```python
from build123d import *

# Parameters (mm, degrees)
F0_R     = 31.9884370587
F1_DEPTH = 25.4


with BuildPart() as f1:
    # F0 (on Front) → F1 (new body)
    with BuildSketch(Plane.XZ):
        Circle(F0_R)
        with BuildLine():
            add(Edge.make_bspline(
                [(-4.1474287559, -5.2462848568), (-2.9695766051, -6.4846808097), (-2.9695766051, -8.3615386761)],
                knots=[0, 0, 0, 1, 1, 1], degree=2))
            add(Edge.make_bspline(
                [(-2.9695766051, -8.3615386761), (-2.9695766051, -10.9924420782), (-4.9289942017, -12.4207254106)],
                knots=[0, 0, 0, 1, 1, 1], degree=2))
            add(Edge.make_bspline(
                [(-4.9289942017, -12.4207254106), (-6.8884117983, -13.8490087429), (-10.4329762146, -13.8490087429)],
                knots=[0, 0, 0, 1, 1, 1], degree=2))
            add(Edge.make_bspline(
                [(-10.4329762146, -13.8490087429), (-14.1811879653, -13.8490087429), (-16.2782051122, -12.6601486281)],
                knots=[0, 0, 0, 1, 1, 1], degree=2))
            Line((-16.2782051122, -12.6601486281), (-16.2782051122, -10.0127332799))
            add(Edge.make_bspline(
                [(-16.2782051122, -10.0127332799), (-14.9187215551, -10.7007310315), (-13.3638466364, -11.0942657455)],
                knots=[0, 0, 0, 1, 1, 1], degree=2))
            add(Edge.make_bspline(
                [(-13.3638466364, -11.0942657455), (-11.8089717178, -11.4878004594), (-10.3614244484, -11.4878004594)],
                knots=[0, 0, 0, 1, 1, 1], degree=2))
            add(Edge.make_bspline(
                [(-10.3614244484, -11.4878004594), (-8.1268077512, -11.4878004594), (-6.9241876814, -10.7750347887)],
                knots=[0, 0, 0, 1, 1, 1], degree=2))
            add(Edge.make_bspline(
                [(-6.9241876814, -10.7750347887), (-5.7215676115, -10.0622691181), (-5.7215676115, -8.5982099026)],
                knots=[0, 0, 0, 1, 1, 1], degree=2))
            add(Edge.make_bspline(
                [(-5.7215676115, -8.5982099026), (-5.7215676115, -7.4974135001), (-6.6737564998, -6.7158480542)],
                knots=[0, 0, 0, 1, 1, 1], degree=2))
            add(Edge.make_bspline(
                [(-6.6737564998, -6.7158480542), (-7.625945388, -5.9342826084), (-10.3999523225, -4.8665100979)],
                knots=[0, 0, 0, 1, 1, 1], degree=2))
            add(Edge.make_bspline(
                [(-10.3999523225, -4.8665100979), (-13.0308557246, -3.8868012996), (-14.1399081002, -3.1547716919)],
                knots=[0, 0, 0, 1, 1, 1], degree=2))
            add(Edge.make_bspline(
                [(-14.1399081002, -3.1547716919), (-15.2489604758, -2.4227420842), (-15.7911027041, -1.495321115)],
                knots=[0, 0, 0, 1, 1, 1], degree=2))
            add(Edge.make_bspline(
                [(-15.7911027041, -1.495321115), (-16.3332449324, -0.5679001459), (-16.3332449324, 0.7200316452)],
                knots=[0, 0, 0, 1, 1, 1], degree=2))
            add(Edge.make_bspline(
                [(-16.3332449324, 0.7200316452), (-16.3332449324, 3.0262001086), (-14.456387066, 4.3609157467)],
                knots=[0, 0, 0, 1, 1, 1], degree=2))
            add(Edge.make_bspline(
                [(-14.456387066, 4.3609157467), (-12.5795291996, 5.6956313848), (-9.3156678659, 5.6956313848)],
                knots=[0, 0, 0, 1, 1, 1], degree=2))
            add(Edge.make_bspline(
                [(-9.3156678659, 5.6956313848), (-6.2719658128, 5.6956313848), (-3.360359328, 4.4572354319)],
                knots=[0, 0, 0, 1, 1, 1], degree=2))
            Line((-3.360359328, 4.4572354319), (-4.3785960004, 2.1345550225))
            add(Edge.make_bspline(
                [(-4.3785960004, 2.1345550225), (-7.213146737, 3.3013992092), (-9.5193152004, 3.3013992092)],
                knots=[0, 0, 0, 1, 1, 1], degree=2))
            add(Edge.make_bspline(
                [(-9.5193152004, 3.3013992092), (-11.5502845632, 3.3013992092), (-12.5822811906, 2.6656892867)],
                knots=[0, 0, 0, 1, 1, 1], degree=2))
            add(Edge.make_bspline(
                [(-12.5822811906, 2.6656892867), (-13.614277818, 2.0299793642), (-13.614277818, 0.9126710156)],
                knots=[0, 0, 0, 1, 1, 1], degree=2))
            add(Edge.make_bspline(
                [(-13.614277818, 0.9126710156), (-13.614277818, 0.1531214978), (-13.2262470861, -0.3780127664)],
                knots=[0, 0, 0, 1, 1, 1], degree=2))
            add(Edge.make_bspline(
                [(-13.2262470861, -0.3780127664), (-12.8382163542, -0.9091470306), (-11.9795951602, -1.3907454568)],
                knots=[0, 0, 0, 1, 1, 1], degree=2))
            add(Edge.make_bspline(
                [(-11.9795951602, -1.3907454568), (-11.1209739662, -1.8723438829), (-8.6772059525, -2.786004897)],
                knots=[0, 0, 0, 1, 1, 1], degree=2))
            add(Edge.make_bspline(
                [(-8.6772059525, -2.786004897), (-5.3252809066, -4.0078889039), (-4.1474287559, -5.2462848568)],
                knots=[0, 0, 0, 1, 1, 1], degree=2))
        make_face(mode=Mode.SUBTRACT)
        with BuildLine():
            Line((17.4336847166, -13.5022578761), (14.5771180519, -13.5022578761))
            Line((14.5771180519, -13.5022578761), (14.5771180519, -1.3054337356))
            add(Edge.make_bspline(
                [(14.5771180519, -1.3054337356), (14.5771180519, 0.9952307458), (13.5286094785, 2.1318030315)],
                knots=[0, 0, 0, 1, 1, 1], degree=2))
            add(Edge.make_bspline(
                [(13.5286094785, 2.1318030315), (12.480100905, 3.2683753171), (10.2399802258, 3.2683753171)],
                knots=[0, 0, 0, 1, 1, 1], degree=2))
            add(Edge.make_bspline(
                [(10.2399802258, 3.2683753171), (7.2678299388, 3.2683753171), (5.9000904086, 1.6502046053)],
                knots=[0, 0, 0, 1, 1, 1], degree=2))
            add(Edge.make_bspline(
                [(5.9000904086, 1.6502046053), (4.5323508784, 0.0320338936), (4.5323508784, -3.644626091)],
                knots=[0, 0, 0, 1, 1, 1], degree=2))
            Line((4.5323508784, -3.644626091), (4.5323508784, -13.5022578761))
            Line((4.5323508784, -13.5022578761), (1.6757842138, -13.5022578761))
            Line((1.6757842138, -13.5022578761), (1.6757842138, 13.2636066525))
            Line((1.6757842138, 13.2636066525), (4.5323508784, 13.2636066525))
            Line((4.5323508784, 13.2636066525), (4.5323508784, 5.1617451295))
            add(Edge.make_bspline(
                [(4.5323508784, 5.1617451295), (4.5323508784, 3.6976859141), (4.3947513281, 2.7344890619)],
                knots=[0, 0, 0, 1, 1, 1], degree=2))
            Line((4.3947513281, 2.7344890619), (4.5653747705, 2.7344890619))
            add(Edge.make_bspline(
                [(4.5653747705, 2.7344890619), (5.4074840185, 4.0939726191), (6.9651109281, 4.8755380649)],
                knots=[0, 0, 0, 1, 1, 1], degree=2))
            add(Edge.make_bspline(
                [(6.9651109281, 4.8755380649), (8.5227378378, 5.6571035107), (10.5151793264, 5.6571035107)],
                knots=[0, 0, 0, 1, 1, 1], degree=2))
            add(Edge.make_bspline(
                [(10.5151793264, 5.6571035107), (13.9716800305, 5.6571035107), (15.7026823736, 4.0141648799)],
                knots=[0, 0, 0, 1, 1, 1], degree=2))
            add(Edge.make_bspline(
                [(15.7026823736, 4.0141648799), (17.4336847166, 2.371226249), (17.4336847166, -1.2063620593)],
                knots=[0, 0, 0, 1, 1, 1], degree=2))
            Line((17.4336847166, -1.2063620593), (17.4336847166, -13.5022578761))
        make_face(mode=Mode.SUBTRACT)
    extrude(amount=F1_DEPTH)


solid = f1.part
```
Here's how the part is built. I have some questions about the finished solid (model axes, mm). A direction names the side the tool comes from. Give positions to 0.01 mm unless a question says otherwise; leave off trailing zeros. Order: outer loops, then holes, each group sorted by start corner. A loop starts at its lowest first (then second) coordinate and runs counter-clockwise, first axis right, second up. Notation, with made-up numbers: (8, 79.25) - (15, 79.25) arc R22 ccw to (15, 99.25) - close; hole circle Ø2 at (63.5, -11). An arc over 180 degrees is marked (long way). Answer as a JSON object with one key per item and string values. Group by question number.
Item 1: If we section it at D-D on x = -19: Please give me the cut outline in (y, z).
Item 2: If we section it at B-B on y = -19: Give the number of separate pieces and of enclosed holes in the cut face, and give its area (3 significant figures).
Item 3: Please list where these lines run through material, in increasing order: probe 1 along X at (y, z) = (-2, -9); probe 2 along Z at (x, y) = (-4, -3.75); probe 3 along Z at (x, y) = (-1, -7.75).
Item 4: If we section it at C-C on z = 19: Please give me the cut outline in (x, y), and give its area (3 significant figures).
Item 5: For P1, Ø6.5, axis at y = -15, z = 8, coming from the -X side; P2, Ø3, axis at x = -1, y = -3, coming from the +Z side; P3, Ø8, axis at x = -19, y = -13, coming from the -Z side, each with a flat end and sliding along its axis, tell me the tip position at first contact or that it passes through.
Item 6: If we mould it in two halves opening along Z, with no side actions, what happens to faces 3 (the flat face through (-4, -13, 3)), 4 (the cylindrical face through (-6.93, -12.52, -31.23)), 5 (the flat face through (0, -25.4, 0))? For each: pulls with the +Z half, pulls with the -Z half, needs draft (parallel to the pull), parting line crosses it, or undercut.
Item 7: Which directions (+Z, -Z, +X, -X, +Y, -Y) give clear straight access to the entire face, cutting with the end or side of a thin tool? Please do faces 1 (the flat face through (0, 0, 0)), 2 (the flat face through (3, -13, -13.502)).
Item 8: If we section it at A-A on z = 8: Please give me the cut outline in (x, y), and give its area (3 significant figures).
Result set:
{
 "1": {"outline": "(-25.4, -25.73) - (0, -25.73) - (0, 25.73) - (-25.4, 25.73) - close"},
 "2": {"separate pieces": "1", "enclosed holes": "2", "area": "2,950 mm²"},
 "3": {"probe 1": "-30.7 to -5.75, -3 to 1.68, 4.53 to 14.58, 17.43 to 30.7", "probe 2": "-31.74 to -11.54, -5.41 to 3, 4.71 to 31.74", "probe 3": "-31.97 to 31.97"},
 "4": {"outline": "(-25.73, -25.4) - (25.73, -25.4) - (25.73, 0) - (-25.73, 0) - close", "area": "1,310 mm²"},
 "5": {"P1": "x = -31.63", "P2": "z = 31.99", "P3": "z = -28.25"},
 "6": {"face 3": "undercut", "face 4": "parting line crosses it", "face 5": "needs draft"},
 "7": {"face 1": "+Z, -Z, +X, -X, +Y", "face 2": "+Y, -Y"},
 "8": {"outline": "(-30.97, -25.4) - (1.68, -25.4) - (1.68, 0) - (-30.97, 0) - close; (4.53, -25.4) - (30.97, -25.4) - (30.97, 0) - (4.53, 0) - close", "area": "1,500 mm²"}
}
